from build123d import *

# Parameters (mm, degrees)
BOSS_EXTRUDE1_DEPTH = 12.1
SKETCH2_R           = 1.25
BOSS_EXTRUDE2_DEPTH = 6.1
CHAMFER1_SIZE       = 0.25
SKETCH3_R           = 1.25
CUT_EXTRUDE1_DEPTH  = 10


with BuildPart() as part:
    # Sketch1 → Boss-Extrude1 (new body)
    with BuildSketch(Plane(origin=(0, 0, 0), x_dir=(1, 0, 0), z_dir=(0, 1, 0))):
        Polygon((2.713546265, 0), (1.356773133, 2.35), (-1.356773133, 2.35), (-2.713546265, 0), (-1.356773133, -2.35), (1.356773133, -2.35), align=None)
    extrude(amount=BOSS_EXTRUDE1_DEPTH)

    # Sketch2 → Boss-Extrude2 (add)
    with BuildSketch(Plane(origin=(0, 12.1, 0), x_dir=(1, 0, 0), z_dir=(0, 1, 0))):
        with Locations(Location((0, 0, 0), (0, 0, 270))):
            Circle(SKETCH2_R)
    extrude(amount=BOSS_EXTRUDE2_DEPTH)

    # Chamfer1
    chamfer1_edges = [part.edges().sort_by_distance(p)[0] for p in [
        (0, 18.2, -1.25),
    ]]
    chamfer(chamfer1_edges, length=CHAMFER1_SIZE)

    # Sketch3 → Cut-Extrude1 (cut)
    with BuildSketch(Plane.XZ):
        with Locations(Location((0, 0, 0), (0, 0, 90))):
            Circle(SKETCH3_R)
    extrude(amount=-CUT_EXTRUDE1_DEPTH, mode=Mode.SUBTRACT)


solid = part.part
Could you check a few things on this model? Use its own coordinates, in mm. A direction names the side the tool comes from. Give positions to 0.01 mm unless a question says otherwise; leave off trailing zeros. Order: outer loops, then holes, each group sorted by start corner. A loop starts at its lowest first (then second) coordinate and runs counter-clockwise, first axis right, second up.
1. For faces 4 (the cylindrical face through (1.22, 4.93, -0.27)), 5 (the flat face through (-2.026, 5.965, -1.191)), 6 (the flat face through (1, 12.1, -1)), which set-ups out of +Z, -Z, +X, -X, +Y, -Y let a thin tool reach every point of the face, with its end or its side?
2. I need wall thicknesses on L1, parallel to Y at x = 1.3, z = 2.1; L2, parallel to Y at x = -0.1, z = -0.05; L3, parallel to Z at x = -1.05, y = 9. Which ranges of each line are inside material? Lowest first, please.
3. We'd pull the mould along Z, two halves only. Please class faces 1 (the flat face through (2.045, 5.965, -1.159)), 2 (the flat face through (2.026, 5.965, 1.191)), 3 (the flat face through (0, 10, 0)): pulls with the +Z half, pulls with the -Z half, needs draft (parallel to the pull), parting line crosses it, or undercut.
4. Suppose I cut it at A-A (y = 4.25). List the corners of the cut face in (x, z) for me, plus the area to 3 significant figures.
5. Will these pins go through, and if not, where does the flat tip stop? P1, Ø1.4, axis at x = -1, z = -0.5, coming from the +Y side; P2, Ø3, axis at x = -1, y = 15.5, coming from the +Z side.
6. Suppose I cut it at D-D (y = 15.5). List the corners of the cut face in (x, z) for me, plus the area to 3 significant figures.
7. Suppose I cut it at B-B (x = 0). List the corners of the cut face in (y, z) for me.
8. Suppose I cut it at C-C (z = -1.75). List the corners of the cut face in (x, y) for me.
Solved:
1. face 4: -Y
1. face 5: -Z, -X, +Y, -Y
1. face 6: +Y
2. L1: y = 0 to 12.1
2. L2: y = 10 to 18.2
2. L3: z = -2.35 to -0.68, 0.68 to 2.35
3. face 1: pulls with the -Z half
3. face 2: pulls with the +Z half
3. face 3: undercut
4. outline: (-2.71, 0) - (-1.36, -2.35) - (1.36, -2.35) - (2.71, 0) - (1.36, 2.35) - (-1.36, 2.35) - close; hole circle Ø2.5 at (0, 0)
4. area: 14.2 mm2
5. P1: stops at y = 18.2
5. P2: stops at z = 1.25
6. outline: circle Ø2.5 at (0, 0)
6. area: 4.91 mm2
7. outline: (0, -2.35) - (12.1, -2.35) - (12.1, -1.25) - (17.95, -1.25) - (18.2, -1) - (18.2, 1) - (17.95, 1.25) - (12.1, 1.25) - (12.1, 2.35) - (0, 2.35) - (0, 1.25) - (10, 1.25) - (10, -1.25) - (0, -1.25) - close
8. outline: (-1.7, 0) - (1.7, 0) - (1.7, 12.1) - (-1.7, 12.1) - close
